Input: part model. Units: mm. Frame: model coordinates. Face numbers are marked on the shaded views. Coordinates: 2 decimals unless noted, no trailing zeros. Write each loop counter-clockwise with the first axis right and the second up, starting at its lowest first coordinate (ties: lowest second). Pieces come first, ordered by that corner, then holes. Notation, with made-up numbers: (-1, -5.5) -> (6, -5.5) arc R34 cw to (6, 25.5) -> close; hole circle Ø11 at (39.5, 47). An arc over 180 degrees is marked (long way). Use one line per item in the form item = value. Start each with the question number.
(1) Pull-direction query (X, two-part tool) for the marked faces 1, 2, 3 and 4; classes: released by +X, released by -X, zero draft, split by the parting line, or undercut.
(2) Cut plane D-D on z = 0. Return the cut outline in (x, y), plus the area to 3 significant figures.
(3) Cut plane C-C on z = 8. Return the cut outline in (x, y).
(4) Cut plane A-A on x = 0. Return the cut outline in (y, z).
(5) Cut plane B-B on y = 1.6. State how many separate pieces and enclosed holes the cut face has, plus the area to 3 significant figures.
(6) Ray query, line 1 along X through (y, z) = (2.05, 0); line 2 along X through (y, z) = (1.85, -5); line 3 along X through (y, z) = (2.15, -4.5). Return the intervals inside material, ascending.
```python
from build123d import *

# Parameters (mm, degrees)
SKETCH_1_R      = 1.6
SKETCH_1_R_2    = 5.5
EXTRUDE_1_DEPTH = 3


with BuildPart() as part:
    # 草图1 → 凸台-拉伸1 (new body)
    with BuildSketch(Plane(origin=(0, 0, 0), x_dir=(1, 0, 0), z_dir=(0, 1, 0))):
        Polygon((-21, 3), (-13, 11), (13, 11), (21, 3), (21, -3), (13, -11), (-13, -11), (-21, -3), align=None)
        with Locations(Location((0, 8, 0), (0, 0, 270))):
            Circle(SKETCH_1_R, mode=Mode.SUBTRACT)
        with Locations(Location((8, 0, 0), (0, 0, 270))):
            Circle(SKETCH_1_R, mode=Mode.SUBTRACT)
        with Locations(Location((-8, 0, 0), (0, 0, 90))):
            Circle(SKETCH_1_R, mode=Mode.SUBTRACT)
        with Locations(Location((0, 0, 0), (0, 0, 270))):
            Circle(SKETCH_1_R_2, mode=Mode.SUBTRACT)
        with Locations(Location((0, -8, 0), (0, 0, 90))):
            Circle(SKETCH_1_R, mode=Mode.SUBTRACT)
        with Locations(Location((-18, 0, 0), (0, 0, 270))):
            Circle(SKETCH_1_R, mode=Mode.SUBTRACT)
        with Locations(Location((-14, 5, 0), (0, 0, 270))):
            Circle(SKETCH_1_R, mode=Mode.SUBTRACT)
        with Locations(Location((-14, -5, 0), (0, 0, 90))):
            Circle(SKETCH_1_R, mode=Mode.SUBTRACT)
        with Locations(Location((14, -5, 0), (0, 0, 270))):
            Circle(SKETCH_1_R, mode=Mode.SUBTRACT)
        with Locations(Location((18, 0, 0), (0, 0, 90))):
            Circle(SKETCH_1_R, mode=Mode.SUBTRACT)
        with Locations(Location((14, 5, 0), (0, 0, 90))):
            Circle(SKETCH_1_R, mode=Mode.SUBTRACT)
    extrude(amount=EXTRUDE_1_DEPTH)


solid = part.part
```
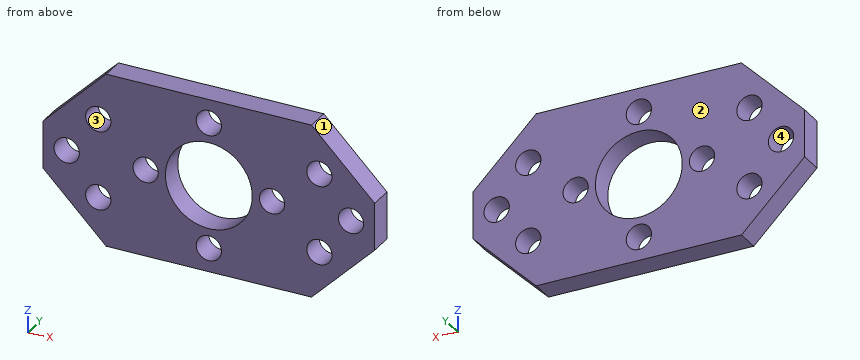
Values:
q1.face_1 = released by +X
q1.face_2 = zero draft
q1.face_3 = undercut
q1.face_4 = undercut
q2.outline = (-21, 0) -> (-19.6, 0) -> (-19.6, 3) -> (-21, 3) -> close; (-16.4, 0) -> (-9.6, 0) -> (-9.6, 3) -> (-16.4, 3) -> close; (-6.4, 0) -> (-5.5, 0) -> (-5.5, 3) -> (-6.4, 3) -> close; (5.5, 0) -> (6.4, 0) -> (6.4, 3) -> (5.5, 3) -> close; (9.6, 0) -> (16.4, 0) -> (16.4, 3) -> (9.6, 3) -> close; (19.6, 0) -> (21, 0) -> (21, 3) -> (19.6, 3) -> close
q2.area = 54.6 mm2
q3.outline = (-16, 0) -> (-1.6, 0) -> (-1.6, 3) -> (-16, 3) -> close; (1.6, 0) -> (16, 0) -> (16, 3) -> (1.6, 3) -> close
q4.outline = (0, -11) -> (3, -11) -> (3, -9.6) -> (0, -9.6) -> close; (0, -6.4) -> (3, -6.4) -> (3, -5.5) -> (0, -5.5) -> close; (0, 5.5) -> (3, 5.5) -> (3, 6.4) -> (0, 6.4) -> close; (0, 9.6) -> (3, 9.6) -> (3, 11) -> (0, 11) -> close
q5.separate_pieces = 1
q5.enclosed_holes = 11
q5.area = 621 mm2
q6.line_1 = -21 to -19.6, -16.4 to -9.6, -6.4 to -5.5, 5.5 to 6.4, 9.6 to 16.4, 19.6 to 21
q6.line_2 = -19 to -15.6, -12.4 to -2.29, 2.29 to 12.4, 15.6 to 19
q6.line_3 = -19.5 to -15.52, -12.48 to -3.16, 3.16 to 12.48, 15.52 to 19.5
